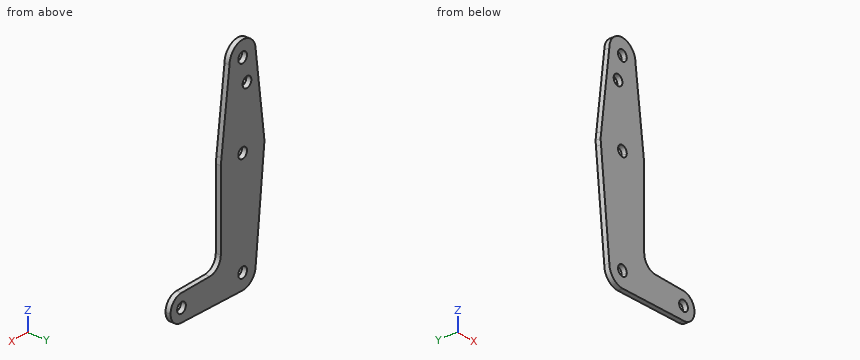
from build123d import *

# Parameters (mm, degrees)
F0_R     = 3.175
F1_DEPTH = 3.048


with BuildPart() as f1:
    # F0 (on Front) → F1 (new body)
    with BuildSketch(Plane.XZ):
        with BuildLine():
            ThreePointArc((-15.3865384615, 67.4076923077), (-9.7463072395, 76.0309664508), (0, 79.375))
            Line((0, 79.375), (0, 99.886942851))
            Line((0, 99.886942851), (0, 104.775))
            ThreePointArc((0, 104.775), (-6.7351920908, 107.5648079092), (-9.525, 114.3))
            Line((-9.525, 114.3), (-15.3865384615, 67.4076923077))
        make_face()
        with Locations((-3.175, 99.886942851)):
            Circle(F0_R, mode=Mode.SUBTRACT)
        with BuildLine():
            ThreePointArc((0, 79.375), (9.7463072395, 76.0309664508), (15.3865384615, 67.4076923077))
            Line((15.3865384615, 67.4076923077), (9.525, 114.3))
            ThreePointArc((9.525, 114.3), (6.7351920908, 107.5648079092), (0, 104.775))
            Line((0, 104.775), (0, 99.886942851))
            Line((0, 99.886942851), (0, 79.375))
        make_face()
        with BuildLine():
            ThreePointArc((0, 104.775), (6.7351920908, 107.5648079092), (9.525, 114.3))
            ThreePointArc((9.525, 114.3), (0, 123.825), (-9.525, 114.3))
            ThreePointArc((-9.525, 114.3), (-6.7351920908, 107.5648079092), (0, 104.775))
        make_face()
        with BuildLine():
            ThreePointArc((3.175, 114.3), (2.2450640303, 112.0549359697), (0, 111.125))
            ThreePointArc((0, 111.125), (-2.2450640303, 116.5450640303), (3.175, 114.3))
        make_face(mode=Mode.SUBTRACT)
        with BuildLine():
            Line((0, 60.325), (0, 47.625))
            ThreePointArc((0, 47.625), (11.2253201513, 52.2746798487), (15.875, 63.5))
            Line((15.875, 63.5), (15.3865384615, 67.4076923077))
            ThreePointArc((15.3865384615, 67.4076923077), (9.7463072395, 76.0309664508), (0, 79.375))
            Line((0, 79.375), (0, 66.675))
            ThreePointArc((0, 66.675), (2.2450640303, 65.7450640303), (3.175, 63.5))
            ThreePointArc((3.175, 63.5), (2.2450640303, 61.2549359697), (0, 60.325))
        make_face()
        with BuildLine():
            ThreePointArc((-15.5606435644, 60.3564356436), (-10.0526499203, 51.2134278751), (0, 47.625))
            Line((0, 47.625), (0, 60.325))
            ThreePointArc((0, 60.325), (-3.175, 63.5), (0, 66.675))
            Line((0, 66.675), (0, 79.375))
            ThreePointArc((0, 79.375), (-9.7463072395, 76.0309664508), (-15.3865384615, 67.4076923077))
            Line((-15.3865384615, 67.4076923077), (-15.875, 63.5))
            Line((-15.875, 63.5), (-15.5606435644, 60.3564356436))
        make_face()
        with BuildLine():
            ThreePointArc((-9.525, 0), (-6.7351920908, 6.7351920908), (0, 9.525))
            Line((0, 9.525), (0, 47.625))
            ThreePointArc((0, 47.625), (-10.0526499203, 51.2134278751), (-15.5606435644, 60.3564356436))
            Line((-15.5606435644, 60.3564356436), (-9.525, 0))
        make_face()
        with BuildLine():
            Line((36.5125, 0), (9.525, 0))
            ThreePointArc((9.525, 0), (6.9712901065, -6.4905114784), (0.6794904459, -9.5007324841))
            Line((0.6794904459, -9.5007324841), (44.45, -7.9375))
            ThreePointArc((44.45, -7.9375), (38.8373399243, -5.6126600757), (36.5125, 0))
        make_face()
        with BuildLine():
            ThreePointArc((3.175, 0), (-2.2450640303, -2.2450640303), (0, 3.175))
            Line((0, 3.175), (0, 9.525))
            ThreePointArc((0, 9.525), (-6.7351920908, 6.7351920908), (-9.525, 0))
            ThreePointArc((-9.525, 0), (-6.7351920908, -6.7351920908), (0, -9.525))
            Line((0, -9.525), (0.6794904459, -9.5007324841))
            ThreePointArc((0.6794904459, -9.5007324841), (6.9712901065, -6.4905114784), (9.525, 0))
            Line((9.525, 0), (3.175, 0))
        make_face()
        with BuildLine():
            Line((0, 47.625), (0, 9.525))
            ThreePointArc((0, 9.525), (6.7351920908, 6.7351920908), (9.525, 0))
            Line((9.525, 0), (36.5125, 0))
            ThreePointArc((36.5125, 0), (38.8373399243, 5.6126600757), (44.45, 7.9375))
            Line((44.45, 7.9375), (23.8252, 7.9375))
            ThreePointArc((23.8252, 7.9375), (18.2035596682, 10.2660596682), (15.875, 15.8877))
            Line((15.875, 15.8877), (15.875, 63.5))
            ThreePointArc((15.875, 63.5), (11.2253201513, 52.2746798487), (0, 47.625))
        make_face()
        with BuildLine():
            Line((0, 9.525), (0, 3.175))
            ThreePointArc((0, 3.175), (2.2450640303, 2.2450640303), (3.175, 0))
            Line((3.175, 0), (9.525, 0))
            ThreePointArc((9.525, 0), (6.7351920908, 6.7351920908), (0, 9.525))
        make_face()
        with BuildLine():
            ThreePointArc((44.45, 7.9375), (38.8373399243, 5.6126600757), (36.5125, 0))
            ThreePointArc((36.5125, 0), (38.8373399243, -5.6126600757), (44.45, -7.9375))
            ThreePointArc((44.45, -7.9375), (50.0626600757, -5.6126600757), (52.3875, 0))
            ThreePointArc((52.3875, 0), (50.0626600757, 5.6126600757), (44.45, 7.9375))
        make_face()
        with BuildLine():
            ThreePointArc((47.625, 0), (44.45, -3.175), (41.275, 0))
            ThreePointArc((41.275, 0), (44.45, 3.175), (47.625, 0))
        make_face(mode=Mode.SUBTRACT)
    extrude(amount=F1_DEPTH)


solid = f1.part
Design review of the part built by this model. Coordinates are the model's own, in mm. Give positions to 0.01 mm unless a question says otherwise; leave off trailing zeros. Loops run counter-clockwise (first coordinate to the right, second up) from the corner with the lowest first, then second, coordinate; pieces in that order, holes last. Notation, with made-up numbers: M 37.5,39 L 89.5,39 A18 ccw 89.5,48 Z; hole C -17.5,79 d8. An arc over 180 degrees is marked long. One line per question, with ' | ' between items. Start each with the question number.
1. Add section C-C (z = 79.5). Write out the cut boundary in (x, y) (3 decimals), plus the area to 3 significant figures.
2. Add section B-B (y = -2.3). Give the number of separate pieces and of enclosed holes in the cut face, plus the area to 3 significant figures.
3. To check wall thickness, follow L1, parallel to X at y = -2.1, z = 114.3 (3 decimals); L2, parallel to X at y = -0.25, z = 2.5 (3 decimals); L3, parallel to X at y = -1.15, z = 62 (3 decimals). State the ranges of each line that lie inside material, in increasing order.
4. Insertion check: P1, Ø0.9, axis at y = -1.5, z = 47.5, coming from the +X side (3 decimals); P2, Ø5.5, axis at x = 0, z = 0, coming from the -Y side; P3, Ø1.5, axis at x = 31, y = -1, coming from the +Z side; P4, Ø1, axis at x = 18.5, y = -1.5, coming from the +Z side. Each pin has a flat end and moves straight along its axis. Give the tip position at first contact, or say it passes through.
5. Add section A-A (x = -5). Write out the cut boundary in (y, z), plus the area to 3 significant figures.
6. Add section D-D (x = 37). Write out the cut boundary in (y, z).
Worked out:
1) outline: M -13.875,-3.048 L 13.875,-3.048 L 13.875,0 L -13.875,0 Z | area: 84.6 mm²
2) separate pieces: 1 | enclosed holes: 5 | area: 3,890 mm²
3) L1: x = -9.525 to -3.175, 3.175 to 9.525 | L2: x = -9.775 to -1.957, 1.957 to 42.493, 46.407 to 51.984 | L3: x = -15.725 to -2.798, 2.798 to 15.875
4) P1: stops at x = 15.875 | P2: passes through | P3: stops at z = 7.94 | P4: stops at z = 10.48
5) outline: M -3.05,-8.11 L 0,-8.11 L 0,97.29 L -3.05,97.29 Z; M -3.05,102.49 L 0,102.49 L 0,122.41 L -3.05,122.41 Z | area: 382 mm²
6) outline: M -3.05,-8.2 L 0,-8.2 L 0,7.94 L -3.05,7.94 Z
